Print and shaded views of the part. All mm, measured from the part's lowest x, y and z. A direction names the side the tool comes from. Coordinates: 2 decimals unless noted, no trailing zeros. Order: outer loops, then holes, each group sorted by start corner. A loop starts at its lowest first (then second) coordinate and runs counter-clockwise, first axis right, second up. Notation, with made-up numbers: M 57,47.25 L 89,47.25 A27 cw 89,70.25 Z; hole C 11,3 d1. An arc over 180 degrees is marked long. Use a Markdown table: item, result. Add a question column.
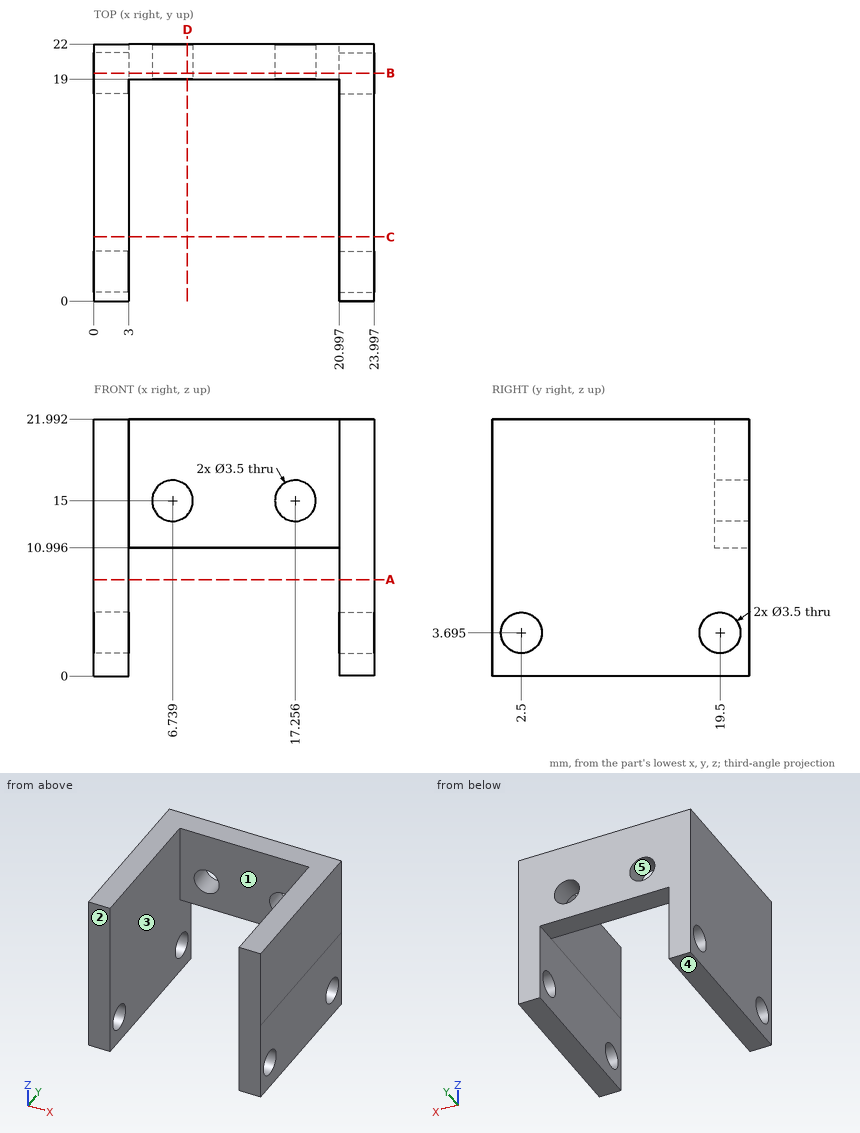
(1) Drop flat-ended pins along their axis: P1, Ø4, axis at x = 16.5, z = 10, coming from the -Y side; P2, Ø3, axis at y = 19.5, z = 3.69, coming from the +X side; P3, Ø1.5, axis at x = 13.5, y = 21, coming from the -Z side. Give the stop position or say it passes through.
(2) Slice it at C-C on y = 5.5. Give the cut face in (x, z), and give its area (3 significant figures).
(3) Slice it at A-A on z = 8.25. Give the cut face in (x, y), and give its area (3 significant figures).
(4) Slice it at B-B on y = 19.5. State how many separate pieces and enclosed holes the cut face has.
(5) Which spindle directions (+Z, -Z, +X, -X, +Y, -Y) get a long thin tool onto all of the face, cutting with end or side? Do the marked faces 1 and 2. Say none if no direction does.
(6) Drill centre lines: line 1 along X through (y, z) = (2.25, 20.25); line 2 along Y through (x, z) = (22, 4.25); line 3 along Y through (x, z) = (12.75, 13.75). Where is each one in solid material? Low to high. Write a range as from..to.
(7) Slice it at D-D on x = 8. Give the cut face in (y, z).
(8) Mould opens along Z. For the marked faces 3, 4 and 5 say: released by +Z, released by -Z, zero draft, split by the parting line, or undercut.
Solutions:
| question | item | result |
|---|---|---|
| 1 | P1 | y = 19 |
| 1 | P2 | through |
| 1 | P3 | z = 11 |
| 2 | outline | M 0,0 L 3,0 L 3,21.99 L 0,21.99 Z; M 21,0 L 24,0 L 24,21.99 L 21,21.99 Z |
| 2 | area | 132 mm² |
| 3 | outline | M 0,0 L 3,0 L 3,22 L 0,22 Z; M 21,0 L 24,0 L 24,22 L 21,22 Z |
| 3 | area | 132 mm² |
| 4 | separate pieces | 3 |
| 4 | enclosed holes | 2 |
| 5 | face 1 | +Z, -Z, -Y |
| 5 | face 2 | +Z, -Z, +X, -X, -Y |
| 6 | line 1 | 0..3, 21..24 |
| 6 | line 2 | 0..0.84, 4.16..17.84, 21.16..22 |
| 6 | line 3 | 19..22 |
| 7 | outline | M 19,11 L 22,11 L 22,13.79 L 19,13.79 Z; M 19,16.21 L 22,16.21 L 22,21.99 L 19,21.99 Z |
| 8 | face 3 | zero draft |
| 8 | face 4 | released by -Z |
| 8 | face 5 | undercut |
